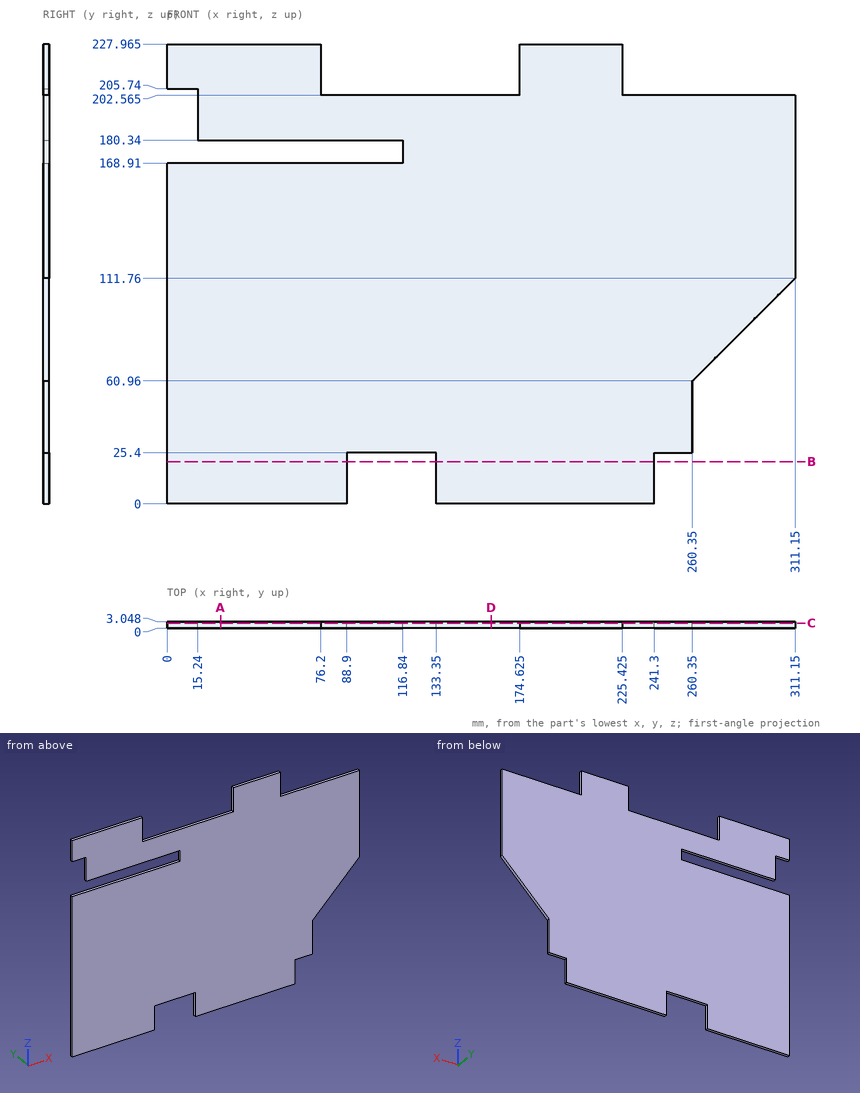
Study the drawing (mm; zero at the part's minimum x, y, z) and answer. Give positions to 0.01 mm unless a question says otherwise; leave off trailing zeros. Write each loop counter-clockwise with the first axis right and the second up, starting at its lowest first coordinate (ties: lowest second). Pieces come first, ordered by that corner, then holes.
(1) The part is cut by section B-B on z = 21. Write down the section's boundary in (x, y), plus the area to 3 significant figures.
Final values:
outline: (0, 0) - (88.9, 0) - (88.9, 3.05) - (0, 3.05) - close; (133.35, 0) - (241.3, 0) - (241.3, 3.05) - (133.35, 3.05) - close
area: 600 mm2
(2) The part is cut by section D-D on x = 160.5. Write down the section's boundary in (y, z) (3 decimals), plus the area to 3 significant figures.
Final values:
outline: (0, 0) - (3.048, 0) - (3.048, 202.565) - (0, 202.565) - close
area: 617 mm2
(3) Straight lines are drawn through the part: line 1 (Z direction, x = 60, y = 1.1) (3 decimals); line 2 (X direction, y = 1.8, z = 212.5) (3 decimals); line 3 (X direction, y = 2.7, z = 47). For each, find the intervals that lie inside material, in ascending order.
Final values:
line 1: z = 0 to 168.91, 180.34 to 227.965
line 2: x = 0 to 76.2, 174.625 to 225.425
line 3: x = 0 to 260.35
(4) The part is cut by section C-C on y = 2.55. Write down the section's boundary in (x, z) (3 decimals), plus the area to 3 significant figures.
Final values:
outline: (0, 0) - (88.9, 0) - (88.9, 25.4) - (133.35, 25.4) - (133.35, 0) - (241.3, 0) - (241.3, 25.4) - (260.35, 25.4) - (260.35, 60.96) - (311.15, 111.76) - (311.15, 202.565) - (225.425, 202.565) - (225.425, 227.965) - (174.625, 227.965) - (174.625, 202.565) - (76.2, 202.565) - (76.2, 227.965) - (0, 227.965) - (0, 205.74) - (15.24, 205.74) - (15.24, 180.34) - (116.84, 180.34) - (116.84, 168.91) - (0, 168.91) - close
area: 58,500 mm2
(5) The part is cut by section A-A on x = 26.5. Write down the section's boundary in (y, z) (3 decimals).
Final values:
outline: (0, 0) - (3.048, 0) - (3.048, 168.91) - (0, 168.91) - close; (0, 180.34) - (3.048, 180.34) - (3.048, 227.965) - (0, 227.965) - close
(6) Flat-ended cylindrical pins translate along their axes: pin 1 Ø0.9 at (x, y) = (145, 1) entering from +Z (3 decimals); pin 2 Ø0.9 at (y, z) = (1.5, 189.5) entering from -X; pin 3 Ø1.5 at (x, y) = (113.5, 2) entering from -Z. Find the tip coordinate at first contact, or state that the pin passes through.
Final values:
pin 1: stops at z = 202.565
pin 2: stops at x = 15.24
pin 3: stops at z = 25.4
